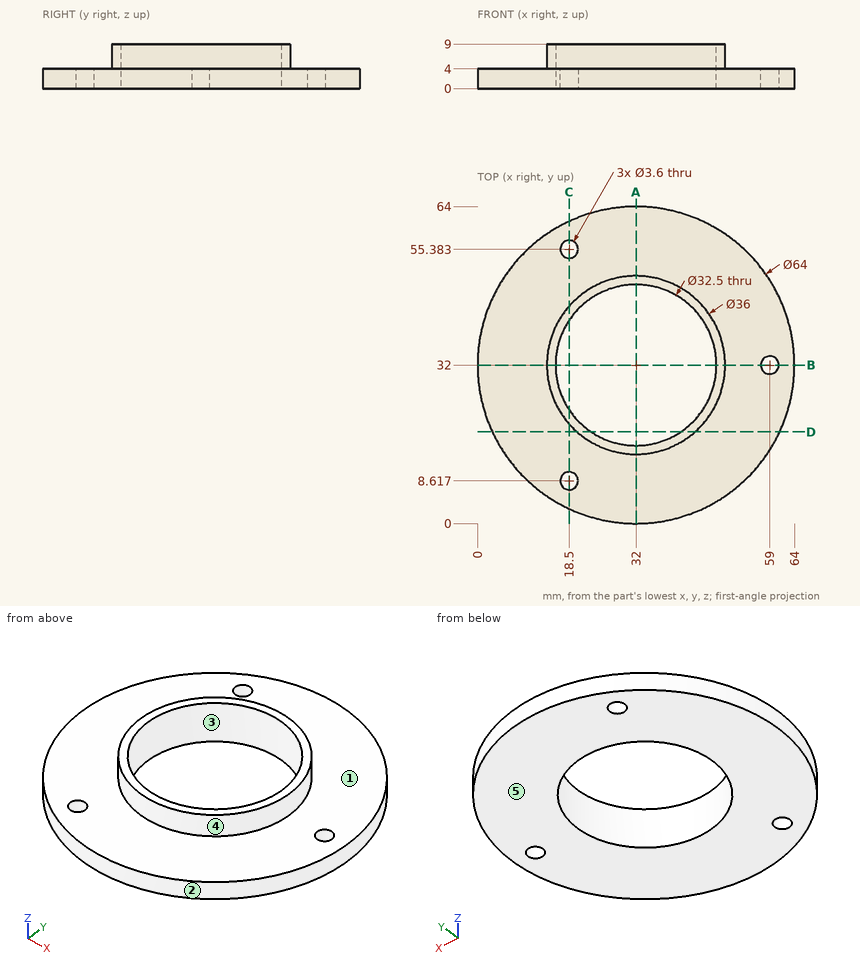
Geometry: see drawing. Coordinates: mm, zero at the bounding-box minimum. A direction names the side the tool comes from. Give positions to 0.01 mm unless a question says otherwise; leave off trailing zeros. Loops run counter-clockwise (first coordinate to the right, second up) from the corner with the lowest first, then second, coordinate; pieces in that order, holes last. Notation, with made-up numbers: (38.25, 82.5) - (66.25, 82.5) arc R19 cw to (66.25, 108.5) - close; hole circle Ø3 at (-39.5, 14.5). An arc over 180 degrees is marked (long way). Answer as CSV lines item,"result". Start each with the question number.
1. Section A-A, the plane x = 32. Return loops of the section in (y, z).
2. Section D-D, the plane y = 18.5. Return loops of the section in (x, z) (1 decimal), plus the area to 3 significant figures.
3. Draft query along X for the marked faces 1, 2 and 3. Return one class per face: released by +X, released by -X, zero draft, split by the parting line, or undercut.
4. Reachability of the marked faces 4 and 5 from +Z, -Z, +X, -X, +Y, -Y: full face, straight path, thin tool, end or side. Return the list, or none.
5. Pin query (flat end, axial travel): P1, Ø6, axis at x = 18.5, y = 8.62, coming from the +Z side; P2, Ø5, axis at y = 18.5, z = 8, coming from the +X side; P3, Ø2, axis at y = 46.5, z = 7, coming from the -X side (1 decimal). Return the tip coordinate at first contact, or that it passes through.
6. Section B-B, the plane y = 32. Return loops of the section in (x, z), plus the area to 3 significant figures.
7. Section C-C, the plane x = 18.5. Return loops of the section in (y, z) (1 decimal).
8. Ray query, L1, parallel to Y at x = 32, z = 2.75; L2, parallel to Z at x = 17, y = 18; L3, parallel to Y at x = 26, z = 8.5. Return the intervals inside material, ascending.
Answers:
1,outline,"(0, 0) - (15.75, 0) - (15.75, 9) - (14, 9) - (14, 4) - (0, 4) - close; (48.25, 0) - (64, 0) - (64, 4) - (50, 4) - (50, 9) - (48.25, 9) - close"
2,outline,"(3, 0) - (23, 0) - (23, 9) - (20.1, 9) - (20.1, 4) - (3, 4) - close; (41, 0) - (61, 0) - (61, 4) - (43.9, 4) - (43.9, 9) - (41, 9) - close"
2,area,"188 mm2"
3,face 1,"zero draft"
3,face 2,"split by the parting line"
3,face 3,"undercut"
4,face 4,"+Z"
4,face 5,"-Z, +X, -X, +Y, -Y"
5,P1,"stops at z = 4"
5,P2,"stops at x = 46.25"
5,P3,"stops at x = 20.1"
6,outline,"(0, 0) - (15.75, 0) - (15.75, 9) - (14, 9) - (14, 4) - (0, 4) - close; (48.25, 0) - (57.2, 0) - (57.2, 4) - (50, 4) - (50, 9) - (48.25, 9) - close; (60.8, 0) - (64, 0) - (64, 4) - (60.8, 4) - close"
6,area,"129 mm2"
7,outline,"(3, 0) - (6.8, 0) - (6.8, 4) - (3, 4) - close; (10.4, 0) - (23, 0) - (23, 9) - (20.1, 9) - (20.1, 4) - (10.4, 4) - close; (41, 0) - (53.6, 0) - (53.6, 4) - (43.9, 4) - (43.9, 9) - (41, 9) - close; (57.2, 0) - (61, 0) - (61, 4) - (57.2, 4) - close"
8,L1,"y = 0 to 15.75, 48.25 to 64"
8,L2,"z = 0 to 4"
8,L3,"y = 15.03 to 16.9, 47.1 to 48.97"
